The model under review builds one solid part; all positions refer to its coordinate system, in mm. A direction names the side the tool comes from. Coordinates: 2 decimals unless noted, no trailing zeros. Write each loop counter-clockwise with the first axis right and the second up, starting at its lowest first coordinate (ties: lowest second). Pieces come first, ordered by that corner, then holes.
```python
from build123d import *

# Parameters (mm, degrees)
SKETCH1_R               = 25
BOSS_EXTRUDE1_DEPTH     = 217
SKETCH2_R               = 19
CUT_EXTRUDE1_DEPTH      = 10
SKETCH3_R               = 14
CUT_EXTRUDE2_DEPTH      = 10
SKETCH4_W               = 43
SKETCH4_H               = 30
CUT_EXTRUDE3_DEPTH      = 26
CUT_EXTRUDE3_DEPTH_BACK = 26
SKETCH5_R               = 8
CUT_EXTRUDE4_DEPTH      = 26
CUT_EXTRUDE4_DEPTH_BACK = 26


with BuildPart() as part:
    # Sketch1 → Boss-Extrude1 (new body)
    with BuildSketch(Plane.XY):
        Circle(SKETCH1_R)
    extrude(amount=BOSS_EXTRUDE1_DEPTH)

    # Sketch2 → Cut-Extrude1 (cut)
    with BuildSketch(Plane(origin=(0, 0, 0), x_dir=(-1, 0, 0), z_dir=(0, 0, -1))):
        Circle(SKETCH2_R)
    extrude(amount=-CUT_EXTRUDE1_DEPTH, mode=Mode.SUBTRACT)

    # Sketch3 → Cut-Extrude2 (cut)
    with BuildSketch(Plane(origin=(0, 0, 10), x_dir=(-1, 0, 0), z_dir=(0, 0, -1))):
        Circle(SKETCH3_R)
    extrude(amount=-CUT_EXTRUDE2_DEPTH, mode=Mode.SUBTRACT)

    # Sketch4 → Cut-Extrude3 (cut, two sides)
    with BuildSketch(Plane(origin=(0, 0, 0), x_dir=(0, 0, -1), z_dir=(1, 0, 0))) as cut_extrude3_sk:
        with Locations((-195.5, 0)):
            Rectangle(SKETCH4_W, SKETCH4_H)
    extrude(amount=CUT_EXTRUDE3_DEPTH, mode=Mode.SUBTRACT)
    extrude(cut_extrude3_sk.sketch, amount=-CUT_EXTRUDE3_DEPTH_BACK, mode=Mode.SUBTRACT)

    # Sketch5 → Cut-Extrude4 (cut, two sides)
    with BuildSketch(Plane(origin=(0, 0, 0), x_dir=(1, 0, 0), z_dir=(0, 1, 0))) as cut_extrude4_sk:
        with Locations((0, -192)):
            Circle(SKETCH5_R)
    extrude(amount=CUT_EXTRUDE4_DEPTH, mode=Mode.SUBTRACT)
    extrude(cut_extrude4_sk.sketch, amount=-CUT_EXTRUDE4_DEPTH_BACK, mode=Mode.SUBTRACT)


solid = part.part
```
Item 1: Take a section at A-A, the plane x = 0. Write out the cut boundary in (y, z), plus the area to 3 significant figures.
Solved:
outline: (-25, 0) - (-19, 0) - (-19, 10) - (-14, 10) - (-14, 20) - (14, 20) - (14, 10) - (19, 10) - (19, 0) - (25, 0) - (25, 184) - (15, 184) - (15, 174) - (-15, 174) - (-15, 184) - (-25, 184) - close; (-25, 200) - (-15, 200) - (-15, 217) - (-25, 217) - close; (15, 200) - (25, 200) - (25, 217) - (15, 217) - close
area: 8,580 mm2
Item 2: Take a section at C-C, the plane z = 192. Write out the cut boundary in (x, y), plus the area to 3 significant figures.
Solved:
outline: (-20, -15) arc R25 ccw to (-8, -23.69) - (-8, -15) - close; (-20, 15) - (-8, 15) - (-8, 23.69) arc R25 ccw to start; (8, -23.69) arc R25 ccw to (20, -15) - (8, -15) - close; (8, 15) - (20, 15) arc R25 ccw to (8, 23.69) - close
area: 253 mm2
Item 3: Machinability: for faces 5 (the face through (0, -15, 201)), 6 (the face through (-12.932, -5.362, 14.93)), 7 (the face through (7.39, 19.94, 195.06)), which of the approach directions +Z, -Z, +X, -X, +Y, -Y give a long, thin tool a straight path to every point of the face, cutting with its end or side? Answer none if there is none.
Solved:
face 5: +Z, +X, -X
face 6: -Z
face 7: +Y, -Y
Item 4: To check wall thickness, follow line 1 along Z through (x, y) = (0, 22); line 2 along Y through (x, z) = (0, 6); line 3 along Y through (x, z) = (-15, 194.5). State the ranges of each line that lie inside material, in increasing order.
Solved:
line 1: z = 0 to 184, 200 to 217
line 2: y = -25 to -19, 19 to 25
line 3: y = -20 to -15, 15 to 20
Item 5: Mouldability with a two-part tool opening along Y and no side actions: class faces 1 (the face through (9, -11, 10)), 2 (the face through (0, 0, 20)), 3 (the face through (-24.976, 1.099, 106.981)), 4 (the face through (-4, 19, 0)) as pulls with the +Y half, pulls with the -Y half, needs draft (parallel to the pull), parting line crosses it, or undercut.
Solved:
face 1: undercut
face 2: undercut
face 3: parting line crosses it
face 4: needs draft
Item 6: Take a section at D-D, the plane y = 0. Write out the cut boundary in (x, z).
Solved:
outline: (-25, 0) - (-19, 0) - (-19, 10) - (-14, 10) - (-14, 20) - (14, 20) - (14, 10) - (19, 10) - (19, 0) - (25, 0) - (25, 174) - (-25, 174) - close
Item 7: Take a section at B-B, the plane y = 17. Write out the cut boundary in (x, z).
Solved:
outline: (-18.33, 0) - (-8.49, 0) - (-8.49, 10) - (8.49, 10) - (8.49, 0) - (18.33, 0) - (18.33, 217) - (-18.33, 217) - close; hole circle Ø16 at (0, 192)
Item 8: For pin 1 (20 mm diameter, centred on x = 3.5, z = 205.5, fed in from -Y); pin 2 (4 mm diameter, centred on x = 1, y = 10, fed in from +Z); pin 3 (2 mm diameter, centred on y = -15.5, z = 154.5, fed in from +X); pin 4 (14 mm diameter, centred on x = 0.5, y = -2.5, fed in from -Z), all flat-tipped, find the tip position at first contact; note any pin that passes through.
Solved:
pin 1: stops at y = -25
pin 2: stops at z = 174
pin 3: stops at x = 20.37
pin 4: stops at z = 20
